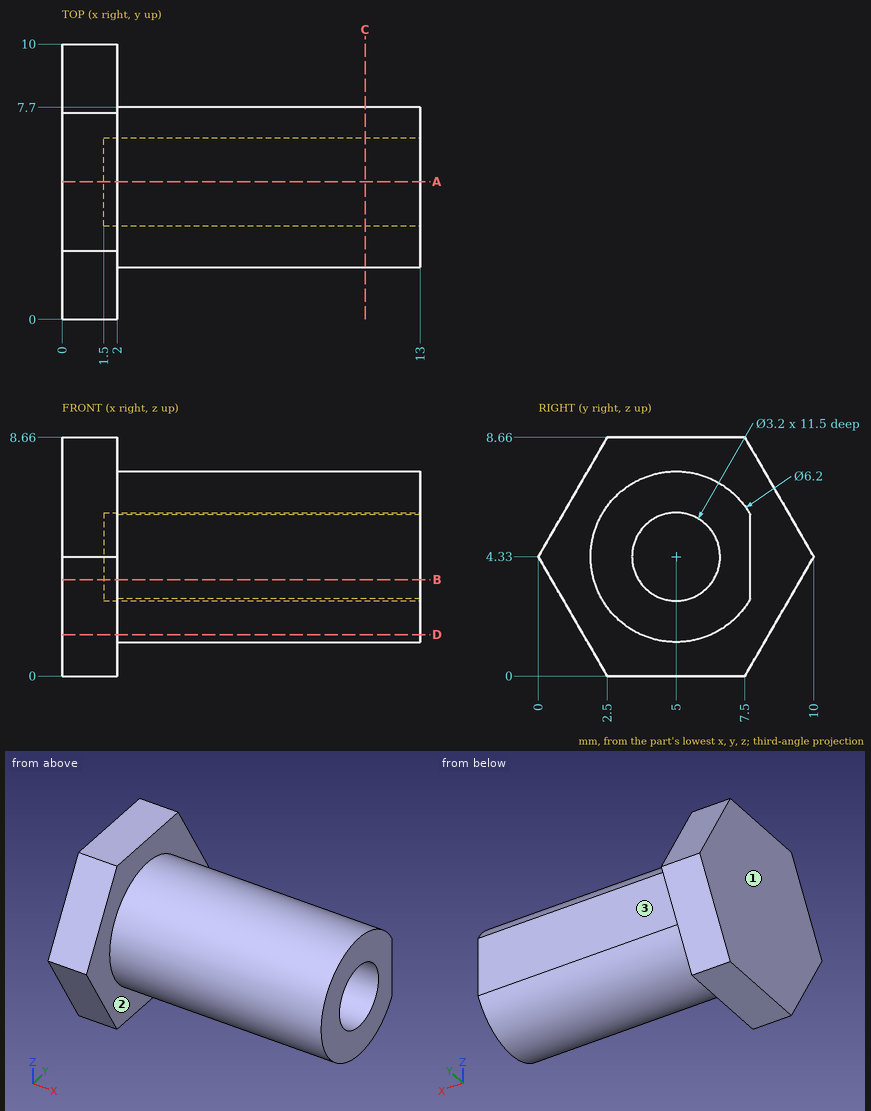
Design review of the part shown in the three views and the two pictorial views. Dimensions are in mm from the part's minimum x, y and z. A direction names the side the tool comes from. Round coordinates to 2 decimals unless told otherwise and drop trailing zeros. Write each loop counter-clockwise with the first axis right and the second up, starting at its lowest first coordinate (ties: lowest second). Pieces come first, ordered by that corner, then holes. Notation, with made-up numbers: (74, 79) -> (97, 79) arc R21 ccw to (97, 115) -> close; hole circle Ø11 at (32, 24). An arc over 180 degrees is marked (long way). Answer as a JSON object with one key per item and string values.
1. We need section D-D on z = 1.5. State the section outline as (x, y) points (1 decimal), and give its area (3 significant figures).
Results found:
{"outline": "(0, 1.6) -> (2, 1.6) -> (2, 3.7) -> (13, 3.7) -> (13, 6.3) -> (2, 6.3) -> (2, 8.4) -> (0, 8.4) -> close", "area": "41.3 mm^2"}
2. We need section C-C on x = 11. State the section outline as (y, z) points.
Results found:
{"outline": "(7.7, 2.81) -> (7.7, 5.85) arc R3.1 ccw (long way) to start; hole circle Ø3.2 at (5, 4.33)"}
3. Machinability: for the marked faces 1, 2 and 3, which of the approach directions +Z, -Z, +X, -X, +Y, -Y give a long, thin tool a straight path to every point of the face, cutting with its end or side? Answer none if there is none.
Results found:
{"face 1": "+Z, -Z, -X, +Y, -Y", "face 2": "+X", "face 3": "+Z, -Z, +X, +Y"}
4. We need section A-A on y = 5. State the section outline as (x, z) points.
Results found:
{"outline": "(0, 0) -> (2, 0) -> (2, 1.23) -> (13, 1.23) -> (13, 2.73) -> (1.5, 2.73) -> (1.5, 5.93) -> (13, 5.93) -> (13, 7.43) -> (2, 7.43) -> (2, 8.66) -> (0, 8.66) -> close"}
5. Clearance check with flat-ended pins moving along their axes: pin 1 (1 mm diameter, centred on y = 5, z = 4.5, fed in from +X); pin 2 (1 mm diameter, centred on x = 1.5, y = 9, fed in from +Z); pin 3 (2.5 mm diameter, centred on x = 5, z = 4, fed in from +Y). State where each tip first meets the part, or that it passes through.
Results found:
{"pin 1": "stops at x = 1.5", "pin 2": "stops at z = 6.93", "pin 3": "stops at y = 7.7"}
6. To check wall thickness, follow line 1 along X through (y, z) = (8, 7.5); line 2 along Y through (x, z) = (3, 2.5); line 3 along X through (y, z) = (4, 5.5). State the ranges of each line that lie inside material, in increasing order.
Results found:
{"line 1": "x = 0 to 2", "line 2": "y = 2.5 to 7.5", "line 3": "x = 0 to 1.5"}
7. We need section B-B on z = 3.5. State the section outline as (x, y) points.
Results found:
{"outline": "(0, 0.48) -> (2, 0.48) -> (2, 2.01) -> (13, 2.01) -> (13, 3.63) -> (1.5, 3.63) -> (1.5, 6.37) -> (13, 6.37) -> (13, 7.7) -> (2, 7.7) -> (2, 9.52) -> (0, 9.52) -> close"}
